Check sheet for the modelled part. Datum: model origin and axes. Units: mm. Face numbers are marked on the shaded views. A direction names the side the tool comes from. Give positions to 0.01 mm unless a question says otherwise; leave off trailing zeros. Write each loop counter-clockwise with the first axis right and the second up, starting at its lowest first coordinate (ties: lowest second). Pieces come first, ordered by that corner, then holes. Notation, with made-up numbers: M 8,33.5 L 64,33.5 A20 ccw 64,56.5 Z; hole C 84.5,-31 d9. An arc over 180 degrees is marked long. Write item = value, one per line. Start each with the question number.
1) Sectioned sample at C-C, the plane x = 33.5. Record the cut outline in (y, z).
2) Sectioned sample at B-B, the plane y = -7.75. Record the cut outline in (x, z), then the cut area to 3 significant figures.
3) Scan lines: L1, parallel to Z at x = 20, y = -7.75; L2, parallel to Z at x = -12.5, y = -3.5; L3, parallel to X at y = -17.75, z = 0. Record each from-to range of solid material in increasing order.
4) Set-up check for the marked faces 1, 2 and 3: record each of +Z, -Z, +X, -X, +Y, -Y from which the full face is reachable in a straight line by a thin tool's end or side.
5) Gauge pin test, flat ends, axial feed: pin 1 (3 mm diameter, centred on x = -34, y = -13.5, fed in from +Z); pin 2 (10 mm diameter, centred on x = 32, y = -14, fed in from -Z); pin 3 (18 mm diameter, centred on x = 20, z = 0, fed in from -Y); pin 4 (12 mm diameter, centred on y = -15.5, z = 1, fed in from +X). Record the tip position at first contact, or that the pin passes through.
6) Sectioned sample at D-D, the plane z = 0. Record the cut outline in (x, y).
7) Sectioned sample at A-A, the plane x = 20. Record the cut outline in (y, z), then the cut area to 3 significant figures.
from build123d import *

# Parameters (mm, degrees)
F1_DEPTH = 25


with BuildPart() as f1:
    # F0 (on Front) → F1 (new body)
    with BuildSketch(Plane.XZ):
        with BuildLine():
            Line((30.154407, 30), (0, 30))
            Line((0, 30), (-30.154407, 30))
            ThreePointArc((-30.154407, 30), (-36.576823, 27.665023), (-40, 21.750515))
            Line((-40, 21.750515), (-40, 7.12132))
            Line((-40, 7.12132), (-37.87868, 5))
            Line((-37.87868, 5), (-28.660254, 5))
            ThreePointArc((-28.660254, 5), (-10, 0), (-28.660254, -5))
            Line((-28.660254, -5), (-37.87868, -5))
            Line((-37.87868, -5), (-40, -7.12132))
            Line((-40, -7.12132), (-40, -21.750515))
            ThreePointArc((-40, -21.750515), (-36.576823, -27.665023), (-30.154407, -30))
            Line((-30.154407, -30), (0, -30))
            Line((0, -30), (30.154407, -30))
            ThreePointArc((30.154407, -30), (36.576823, -27.665023), (40, -21.750515))
            Line((40, -21.750515), (40, -7.12132))
            Line((40, -7.12132), (37.87868, -5))
            Line((37.87868, -5), (28.660254, -5))
            ThreePointArc((28.660254, -5), (10, 0), (28.660254, 5))
            Line((28.660254, 5), (37.87868, 5))
            Line((37.87868, 5), (40, 7.12132))
            Line((40, 7.12132), (40, 21.750515))
            ThreePointArc((40, 21.750515), (36.576823, 27.665023), (30.154407, 30))
        make_face()
    extrude(amount=F1_DEPTH)


solid = f1.part
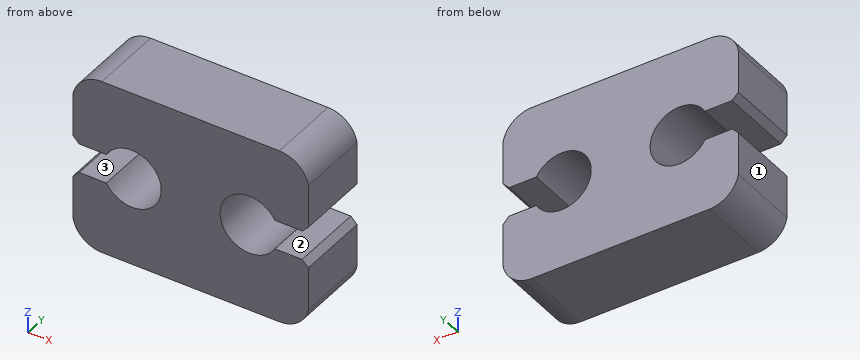
Data:
q1.outline = M -25,-29.42 L 0,-29.42 L 0,-5 L -25,-5 Z; M -25,5 L 0,5 L 0,29.42 L -25,29.42 Z
q2.outline = M -40,-21.75 A10 ccw -30.15,-30 L 30.15,-30 A10 ccw 40,-21.75 L 40,-7.12 L 37.88,-5 L 28.66,-5 A10 cw long 28.66,5 L 37.88,5 L 40,7.12 L 40,21.75 A10 ccw 30.15,30 L -30.15,30 A10 ccw -40,21.75 L -40,7.12 L -37.88,5 L -28.66,5 A10 cw long -28.66,-5 L -37.88,-5 L -40,-7.12 Z
q2.area = 3,870 mm2
q3.L1 = -30 to -10, 10 to 30
q3.L2 = -30 to -6.61, 6.61 to 30
q3.L3 = -10 to 10
q4.face_1 = +Z, -Z, -X, +Y, -Y
q4.face_2 = +X, +Y, -Y
q4.face_3 = -X, +Y, -Y
q5.pin_1 = 29.72
q5.pin_2 = -30
q5.pin_3 = through
q5.pin_4 = 39.88
q6.outline = M -10,-25 L 10,-25 L 10,0 L -10,0 Z
q7.outline = M -25,-30 L 0,-30 L 0,-10 L -25,-10 Z; M -25,10 L 0,10 L 0,30 L -25,30 Z
q7.area = 1,000 mm2
